from build123d import *

# Parameters (mm, degrees)
SKETCH1_W               = 207
SKETCH1_H               = 117
BOSS_EXTRUDE1_DEPTH     = 4.5
SKETCH2_R               = 1.5
CUT_EXTRUDE1_DEPTH      = 5.5
MIRROR3_COPY_1_SKETCH_R = 1.5
MIRROR3_COPY_1_DEPTH    = 5.5
CUT_EXTRUDE2_DEPTH      = 4.5


with BuildPart() as part:
    # Sketch1 → Boss-Extrude1 (new body)
    with BuildSketch(Plane.XY):
        Rectangle(SKETCH1_W, SKETCH1_H)
    extrude(amount=BOSS_EXTRUDE1_DEPTH)

    # Sketch2 → Cut-Extrude1 (cut, through all)
    with BuildSketch(Plane.XY.offset(4.5)):
        with Locations((-77.5, 44)):
            Circle(SKETCH2_R)
    cut_extrude1 = extrude(amount=-CUT_EXTRUDE1_DEPTH, mode=Mode.SUBTRACT)

    # Mirror1: Cut-Extrude1 across plane
    add(cut_extrude1.mirror(Plane(origin=(0, 0, 0), x_dir=(0, 0, 1), z_dir=(1, 0, 0))), mode=Mode.SUBTRACT)

    # Mirror3: Cut-Extrude1 across plane
    add(cut_extrude1.mirror(Plane.ZX), mode=Mode.SUBTRACT)

    # Mirror3 copy 1 sketch → Mirror3 copy 1 (cut, through all)
    with BuildSketch(Plane(origin=(0, 0, 4.5), x_dir=(-1, 0, 0), z_dir=(0, 0, 1))):
        with Locations((-77.5, 44)):
            Circle(MIRROR3_COPY_1_SKETCH_R)
    extrude(amount=-MIRROR3_COPY_1_DEPTH, mode=Mode.SUBTRACT)

    # Sketch3 → Cut-Extrude2 (cut)
    with BuildSketch(Plane.XY.offset(4.5)):
        with BuildLine():
            Line((74.50260241, 58.5), (74.041825512, 54.178381356))
            ThreePointArc((74.041825512, 54.178381356), (74.287682649, 53.401965683), (75.025093069, 53.056288231))
            Line((75.025093069, 53.056288231), (103.5, 52.330947596))
            Line((103.5, 52.330947596), (103.5, 58.5))
            Line((103.5, 58.5), (74.50260241, 58.5))
        make_face()
    cut_extrude2 = extrude(amount=-CUT_EXTRUDE2_DEPTH, mode=Mode.SUBTRACT)

    # Mirror4: Cut-Extrude2 across plane
    add(cut_extrude2.mirror(Plane.ZX), mode=Mode.SUBTRACT)


solid = part.part
CAD build for the part. Positions are in the model's coordinates, mm. Coordinates: 2 decimals unless noted, no trailing zeros. Loops run counter-clockwise (first coordinate to the right, second up) from the corner with the lowest first, then second, coordinate; pieces in that order, holes last. Notation, with made-up numbers: (53.25, -34.75) - (65.25, -34.75) arc R8 cw to (65.25, -29.75) - close; hole circle Ø11 at (-18, 10). An arc over 180 degrees is marked (long way). Write item = value, one per line. Start each with the question number.
Q1. Cut at A-A, the plane z = 1.45. List the corners of the cut face in (x, y), then the cut area to 3 significant figures.
Q2. Drill centre lines: L1, parallel to X at y = -44, z = 3.5; L2, parallel to Y at x = -77.5, z = 1.4; L3, parallel to Y at x = 77.5, z = 2.6. Where is each one in solid material? Low to high.
Q3. Pull direction Y, two halves, no side cores. Call faces 1 (the flat face through (-1, 1, 4.5)), 2 (the flat face through (-16, 58.5, 2)), 3 (the flat face through (74.275, -56.369, 2.282)), 4 (the flat face through (74.275, 56.369, 2.282)): pulls with the +Y half, pulls with the -Y half, needs draft (parallel to the pull), parting line crosses it, or undercut.
Computed:
q1.outline = (-103.5, -58.5) - (74.5, -58.5) - (74.04, -54.18) arc R1.01 cw to (75.03, -53.06) - (103.5, -52.33) - (103.5, 52.33) - (75.03, 53.06) arc R1.01 cw to (74.04, 54.18) - (74.5, 58.5) - (-103.5, 58.5) - close; hole circle Ø3 at (-77.5, -44); hole circle Ø3 at (-77.5, 44); hole circle Ø3 at (77.5, -44); hole circle Ø3 at (77.5, 44)
q1.area = 23,900 mm²
q2.L1 = -103.5 to -79, -76 to 76, 79 to 103.5
q2.L2 = -58.5 to -45.5, -42.5 to 42.5, 45.5 to 58.5
q2.L3 = -52.99 to -45.5, -42.5 to 42.5, 45.5 to 52.99
q3.face_1 = needs draft
q3.face_2 = pulls with the +Y half
q3.face_3 = undercut
q3.face_4 = undercut
